Verification items for this drawing (mm, ordinates from the low corner). A direction names the side the tool comes from. Round coordinates to 2 decimals unless told otherwise and drop trailing zeros. Write each loop counter-clockwise with the first axis right and the second up, starting at its lowest first coordinate (ties: lowest second). Pieces come first, ordered by that corner, then holes. Notation, with made-up numbers: M 58.25,-19.75 L 84.25,-19.75 A36 cw 84.25,17.25 Z; hole C 56,67 d11. An arc over 180 degrees is marked long. Write each question's results on one line, items separated by ' | '.
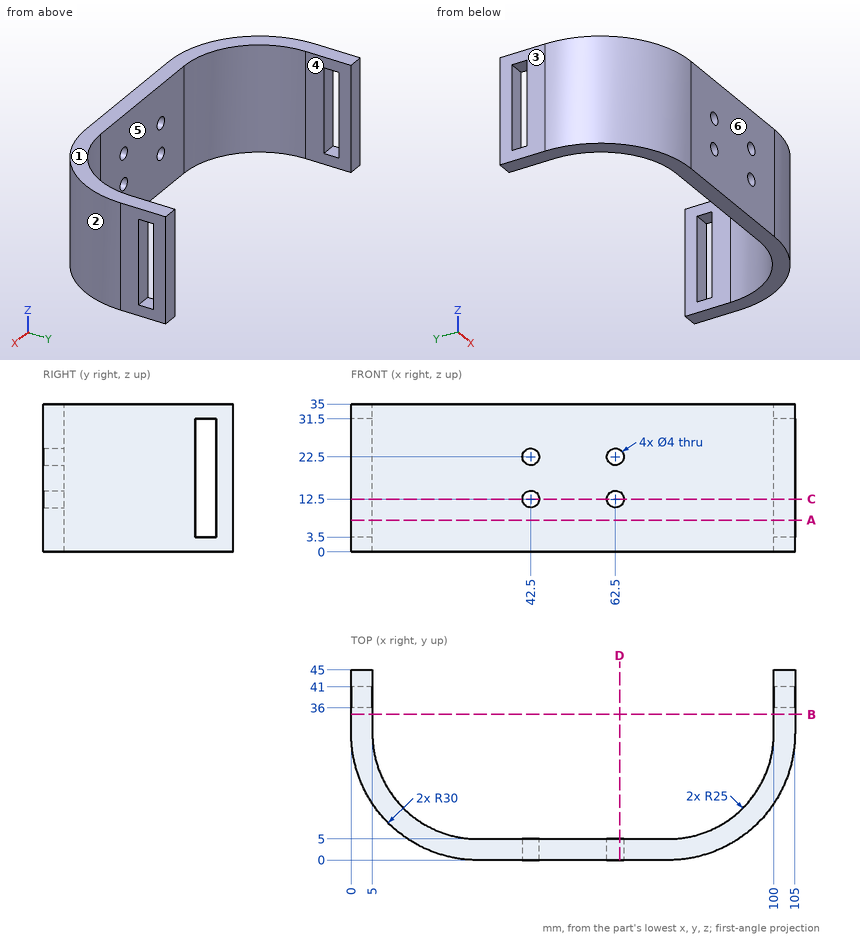
1) Depth check by flat-ended pin: P1, Ø10.5, axis at x = 48.5, z = 10.5, coming from the +Y side; P2, Ø4, axis at y = 10.5, z = 19, coming from the +X side; P3, Ø2.5, axis at x = 1.5, z = 14.5, coming from the -Y side; P4, Ø10, axis at x = 91, y = 27.5, coming from the -Z side. Enter the tip coordinate at first touch or a pass-through.
Calculated:
P1: stops at y = 5 | P2: stops at x = 99.37 | P3: stops at y = 17.45 | P4: passes through
2) Sectioned sample at D-D, the plane x = 63.5. Record the cut outline in (y, z), and give its area (3 significant figures).
Calculated:
outline: M 0,0 L 5,0 L 5,10.77 L 0,10.77 Z; M 0,14.23 L 5,14.23 L 5,20.77 L 0,20.77 Z; M 0,24.23 L 5,24.23 L 5,35 L 0,35 Z | area: 140 mm²
3) Sectioned sample at B-B, the plane y = 34.5. Record the cut outline in (x, z).
Calculated:
outline: M 0,0 L 5,0 L 5,35 L 0,35 Z; M 100,0 L 105,0 L 105,35 L 100,35 Z
4) Sectioned sample at A-A, the plane z = 7.5. Record the cut outline in (x, y).
Calculated:
outline: M 0,30 A30 ccw 30,0 L 75,0 A30 ccw 105,30 L 105,36 L 100,36 L 100,30 A25 cw 75,5 L 30,5 A25 cw 5,30 L 5,36 L 0,36 Z; M 0,41 L 5,41 L 5,45 L 0,45 Z; M 100,41 L 105,41 L 105,45 L 100,45 Z
5) Access from +Z, -Z, +X, -X, +Y, -Y to the whole of each face (thin tool, end or side, straight path). Record for the marked faces 5 and 6.
Calculated:
face 5: +Z, -Z, +Y | face 6: +Z, -Z, +X, -X, -Y
6) Sectioned sample at C-C, the plane z = 12.5. Record the cut outline in (x, y).
Calculated:
outline: M 0,30 A30 ccw 30,0 L 40.5,0 L 40.5,5 L 30,5 A25 cw 5,30 L 5,36 L 0,36 Z; M 0,41 L 5,41 L 5,45 L 0,45 Z; M 44.5,0 L 60.5,0 L 60.5,5 L 44.5,5 Z; M 64.5,0 L 75,0 A30 ccw 105,30 L 105,36 L 100,36 L 100,30 A25 cw 75,5 L 64.5,5 Z; M 100,41 L 105,41 L 105,45 L 100,45 Z
7) Draft check along X on the marked faces 1, 2, 3 and 4. Enter one of: pulls with the +X half, pulls with the -X half, needs draft (parallel to the pull), parting line crosses it, or undercut.
Calculated:
face 1: needs draft | face 2: pulls with the +X half | face 3: pulls with the -X half | face 4: undercut
8) Material ranges on line 1 (X direction, y = 29, z = 5.5); line 2 (Y direction, x = 41.5, z = 6); line 3 (X direction, y = 3, z = 12), recorded low to high. Write a range as [from, to].
Calculated:
line 1: x = [0.02, 5.02], [99.98, 104.98] | line 2: y = [0, 5] | line 3: x = [16.92, 40.56], [44.44, 60.56], [64.44, 88.08]
